Design review of the part built by this model. Coordinates are the model's own, in mm. A direction names the side the tool comes from. Give positions to 0.01 mm unless a question says otherwise; leave off trailing zeros. Loops run counter-clockwise (first coordinate to the right, second up) from the corner with the lowest first, then second, coordinate; pieces in that order, holes last. Notation, with made-up numbers: (-35, 29) - (-28, 29) arc R23 cw to (-28, 53) - close; hole circle Ø1 at (89, 63.25). An arc over 180 degrees is marked (long way). Write each question's results on one line, items separated by ' | '.
from build123d import *
from build123d.topology import SkipClean

# Parameters (mm, degrees)
EXTRUDE_1_DEPTH        = 4
EXTRUDE_3_DEPTH        = 6
CHAMFER_1_SIZE         = 3
SKETCH_5_R             = 0.85
CUT_EXTRUDE_1_DEPTH    = 4
PATTERN_LINEAR_1_COUNT = 4
PATTERN_LINEAR_1_PITCH = 8
CUT_EXTRUDE_2_DEPTH    = 2.5
CUT_EXTRUDE_3_REACH    = 41.439
SKETCH_7_R             = 1.35
SKETCH_8_R             = 6
EXTRUDE_4_DEPTH        = 1.5
FILLET_1_R             = 0.5
SKETCH_9_R             = 5
CUT_EXTRUDE_4_DEPTH    = 3.6
SKETCH_10_R            = 3.55
CUT_EXTRUDE_5_DEPTH    = 3.6
CUT_EXTRUDE_6_DEPTH    = 0.8
CUT_EXTRUDE_7_DEPTH    = 40.958228189
FILLET_2_R             = 2
CHAMFER_2_SIZE         = 1


with BuildPart() as part:
    # ｽｹｯﾁ1 → ﾎﾞｽ - 押し出し1 (new body)
    with BuildSketch(Plane(origin=(0, 0, 0), x_dir=(1, 0, 0), z_dir=(0, 1, 0))):
        with BuildLine():
            Line((-7.9, 0), (-7.9, -38))
            Line((-7.9, -38), (7.9, -38))
            Line((7.9, -38), (7.9, 0))
            ThreePointArc((7.9, 0), (0, 7.9), (-7.9, 0))
        make_face()
    extrude(amount=EXTRUDE_1_DEPTH)

    # ｽｹｯﾁ4 → ﾎﾞｽ - 押し出し3 (add)
    with BuildSketch(Plane.XY.offset(38)):
        Polygon((-7, -5.5), (-4.5, -5.5), (-3, -2), (3, -2), (4.5, -5.5), (7, -5.5), (7.9, -2), (7.9, 0), (-7.9, 0), (-7.9, -2), align=None)
    extrude(amount=-EXTRUDE_3_DEPTH)

    # 面取り1
    chamfer_1_edges = [part.edges().sort_by_distance(p)[0] for p in [
        (0, 4, 38),
    ]]
    chamfer(chamfer_1_edges, length=CHAMFER_1_SIZE)

    # ｽｹｯﾁ5 → ｶｯﾄ - 押し出し1 (cut)
    with BuildSketch(Plane(origin=(0, 4, 0), x_dir=(1, 0, 0), z_dir=(0, 1, 0))):
        with Locations(Location((-4, -31, 0), (0, 0, 270))):
            Circle(SKETCH_5_R)
        with Locations(Location((4, -31, 0), (0, 0, 270))):
            Circle(SKETCH_5_R)
    cut_extrude_1 = extrude(amount=-CUT_EXTRUDE_1_DEPTH, mode=Mode.SUBTRACT)

    # 直線ﾊﾟﾀｰﾝ1: ｶｯﾄ - 押し出し1 ×4
    with Locations(*[(0, 0, -i * PATTERN_LINEAR_1_PITCH) for i in range(1, PATTERN_LINEAR_1_COUNT)]):
        add(cut_extrude_1, mode=Mode.SUBTRACT)

    # ｽｹｯﾁ6 → ｶｯﾄ - 押し出し2 (cut)
    with BuildSketch(Plane(origin=(0, 4, 0), x_dir=(1, 0, 0), z_dir=(0, 1, 0))):
        with BuildLine():
            Line((-3, -35), (-3, -39))
            Line((-3, -39), (3, -39))
            Line((3, -39), (3, -35))
            ThreePointArc((3, -35), (0, -32), (-3, -35))
        make_face()
    extrude(amount=-CUT_EXTRUDE_2_DEPTH, mode=Mode.SUBTRACT)

    # ｽｹｯﾁ7 → ｶｯﾄ - 押し出し3 (cut, up to next)
    with BuildSketch(Plane(origin=(0, 1.5, 0), x_dir=(1, 0, 0), z_dir=(0, 1, 0)), mode=Mode.PRIVATE) as cut_extrude_3_sk1:
        with Locations(Location((0, -35, 0), (0, 0, 270))):
            Circle(SKETCH_7_R)
    cut_extrude_3_tool1 = extrude(cut_extrude_3_sk1.sketch, amount=-CUT_EXTRUDE_3_REACH, mode=Mode.PRIVATE) & part.part
    add(cut_extrude_3_tool1.solids().sort_by_distance((0, 1.5, 35))[0], mode=Mode.SUBTRACT)

    # ｽｹｯﾁ8 → ﾎﾞｽ - 押し出し4 (add)
    with BuildSketch(Plane.XZ):
        with Locations(Location((0, 0, 0), (0, 0, 90))):
            Circle(SKETCH_8_R)
    extrude(amount=EXTRUDE_4_DEPTH)

    # ﾌｨﾚｯﾄ1
    fillet_1_edges = [part.edges().sort_by_distance(p)[0] for p in [
        (0, 0, -6),
    ]]
    fillet(fillet_1_edges, radius=FILLET_1_R)

    # ｽｹｯﾁ9 → ｶｯﾄ - 押し出し4 (cut)
    with BuildSketch(Plane(origin=(0, 4, 0), x_dir=(1, 0, 0), z_dir=(0, 1, 0))):
        with Locations(Location((0, 0, 0), (0, 0, 270))):
            Circle(SKETCH_9_R)
    extrude(amount=-CUT_EXTRUDE_4_DEPTH, mode=Mode.SUBTRACT)

    # ｽｹｯﾁ10 → ｶｯﾄ - 押し出し5 (cut)
    with BuildSketch(Plane(origin=(0, 0.4, 0), x_dir=(1, 0, 0), z_dir=(0, 1, 0))):
        with Locations(Location((0, 0, 0), (0, 0, 270))):
            Circle(SKETCH_10_R)
    extrude(amount=-CUT_EXTRUDE_5_DEPTH, mode=Mode.SUBTRACT)

    # ｽｹｯﾁ11 → ｶｯﾄ - 押し出し6 (cut, symmetric)
    with BuildSketch(Plane.XY.offset(35)):
        Polygon((3, -2), (4.5, -5.5), (5.1, -5.5), (3.6, -2), align=None)
        Polygon((7.9, -2), (7, -5.5), (6.4, -5.5), (7.3, -2), align=None)
    cut_extrude_6 = extrude(amount=CUT_EXTRUDE_6_DEPTH, both=True, mode=Mode.SUBTRACT)

    # ﾐﾗｰ1: ｶｯﾄ - 押し出し6 across plane
    add(cut_extrude_6.mirror(Plane(origin=(0, 0, 0), x_dir=(0, 0, 1), z_dir=(1, 0, 0))), mode=Mode.SUBTRACT)

    # ｽｹｯﾁ12 → ｶｯﾄ - 押し出し7 (cut, through all)
    with SkipClean():  # the faces are left unmerged after this step: merging them gives an invalid solid
        with BuildSketch(Plane(origin=(0, 4, 0), x_dir=(1, 0, 0), z_dir=(0, 1, 0))):
            with BuildLine():
                Line((-7.9, 0), (-7.9, -30))
                Line((-7.9, -30), (-6.9, -27))
                Line((-6.9, -27), (-6.9, -3.847076812))
                ThreePointArc((-6.9, -3.847076812), (-7.645913941, -1.987460691), (-7.9, 0))
            make_face()
        cut_extrude_7 = extrude(amount=-CUT_EXTRUDE_7_DEPTH, mode=Mode.SUBTRACT)

    # ﾐﾗｰ2: ｶｯﾄ - 押し出し7 across plane
    with SkipClean():  # the faces are left unmerged after this step: merging them gives an invalid solid
        add(cut_extrude_7.mirror(Plane(origin=(0, 0, 0), x_dir=(0, 0, 1), z_dir=(1, 0, 0))), mode=Mode.SUBTRACT)

    # ﾌｨﾚｯﾄ2
    fillet_2_edges = [part.edges().sort_by_distance(p)[0] for p in [
        (-6.9, 2, 3.847076812),
        (-6.9, 2, 27),
        (-7.9, 2, 30),
        (6.9, 2, 3.847076812),
        (7.9, 2, 30),
        (6.9, 2, 27),
    ]]
    fillet(fillet_2_edges, radius=FILLET_2_R)

    # 面取り2
    # the kernel refuses this chamfer: 1 mm, written as the material it adds along each edge
    with BuildSketch(Plane(origin=(7.9, 0, 32), x_dir=(0, 0.02749587661058639, -0.9996219169112968), z_dir=(-1, 0, 0))) as chamfer_2_piece_1_section:
        Polygon((CHAMFER_2_SIZE * 0.999621916911, CHAMFER_2_SIZE * 0.0274958766106), (-CHAMFER_2_SIZE * 0.0274958766106, CHAMFER_2_SIZE * 0.999621916911), (0, 0), align=None)
    chamfer_2_piece_1 = extrude(amount=15.8, mode=Mode.PRIVATE)
    chamfer_2_piece_1 = chamfer_2_piece_1 - Plane(origin=(-4, -0.34097177, 31), x_dir=(0, 0, 1), z_dir=(0, 1, 0)) * Cylinder(0.85, 36, mode=Mode.PRIVATE)
    chamfer_2_piece_1 = chamfer_2_piece_1 - Plane(origin=(4, -0.34097177, 31), x_dir=(0, 0, 1), z_dir=(0, 1, 0)) * Cylinder(0.85, 36, mode=Mode.PRIVATE)
    add(chamfer_2_piece_1)
    # the kernel refuses this chamfer: 1 mm, written as the material it takes off along each edge
    with BuildSketch(Plane(origin=(-7.9, 4, 30.32455532), x_dir=(-0.027495876610586487, -0.9996219169112968, 0), z_dir=(0, 0, 1)), Plane(origin=(7.9, 4, 37.571682988), x_dir=(0.027495876610586487, -0.9996219169112968, 0), z_dir=(0, 0, -1))) as chamfer_2_2_piece_1:
        Polygon((CHAMFER_2_SIZE * 0.999621916911, CHAMFER_2_SIZE * 0.0274958766106), (-CHAMFER_2_SIZE * 0.0274958766106, CHAMFER_2_SIZE * 0.999621916911), (0, 0), align=None)
    extrude(amount=7.247127668, mode=Mode.SUBTRACT)
    with BuildSketch(Plane(origin=(0, 4, 0), x_dir=(1, 0, 0), z_dir=(0, 0, 1))) as chamfer_2_2_piece_2:
        Polygon((7.9, -CHAMFER_2_SIZE), (7.9 - CHAMFER_2_SIZE, 0), (7.9, 0), align=None)
    revolve(axis=Axis((0, 4, 0), (0, 1, 0)), revolution_arc=180, mode=Mode.SUBTRACT)
    with BuildSketch(Plane(origin=(-5.9, 4, 30.32455532), x_dir=(-1, 0, 0), z_dir=(0, 0, 1))) as chamfer_2_2_piece_3:
        Polygon((2, CHAMFER_2_SIZE), (2 - CHAMFER_2_SIZE, 0), (2, 0), align=None)
    revolve(axis=Axis((-5.9, 4, 30.32455532), (0, -1, 0)), revolution_arc=18.434948823, mode=Mode.SUBTRACT)
    with BuildSketch(Plane(origin=(-7.797366596, 4, 29.692099788), x_dir=(-0.02608487890572092, -0.9996219169112968, -0.008694959635240314), z_dir=(0.3162277660168382, 0, -0.9486832980505138))) as chamfer_2_2_piece_4:
        Polygon((CHAMFER_2_SIZE * 0.999621916911, -CHAMFER_2_SIZE * 0.0274958766106), (-CHAMFER_2_SIZE * 0.0274958766106, -CHAMFER_2_SIZE * 0.999621916911), (0, 0), align=None)
    extrude(amount=2.513167019, mode=Mode.SUBTRACT)
    with BuildSketch(Plane(origin=(-8.9, 4, 26.67544468), x_dir=(0.9486832980505135, 0, 0.3162277660168389), z_dir=(-0.3162277660168389, 0, 0.9486832980505135))) as chamfer_2_2_piece_5:
        Polygon((2, -CHAMFER_2_SIZE), (2 + CHAMFER_2_SIZE, 0), (2, 0), align=None)
    revolve(axis=Axis((-8.9, 4, 26.67544468), (0, 1, 0)), revolution_arc=18.434948823, mode=Mode.SUBTRACT)
    with BuildSketch(Plane(origin=(-6.9, 4, 26.67544468), x_dir=(-0.027495876610586487, -0.9996219169112968, 0), z_dir=(0, 0, -1))) as chamfer_2_2_piece_6:
        Polygon((CHAMFER_2_SIZE * 0.999621916911, -CHAMFER_2_SIZE * 0.0274958766106), (-CHAMFER_2_SIZE * 0.0274958766106, -CHAMFER_2_SIZE * 0.999621916911), (0, 0), align=None)
    extrude(amount=22.339548002, mode=Mode.SUBTRACT)
    with BuildSketch(Plane(origin=(-8.9, 4, 4.335896678), x_dir=(1, 0, 0), z_dir=(0, 0, 1))) as chamfer_2_2_piece_7:
        Polygon((2, -CHAMFER_2_SIZE), (2 + CHAMFER_2_SIZE, 0), (2, 0), align=None)
    revolve(axis=Axis((-8.9, 4, 4.335896678), (0, 1, 0)), revolution_arc=25.974390018, mode=Mode.SUBTRACT)
    with BuildSketch(Plane(origin=(8.9, 4, 4.335896678), x_dir=(-0.8989898989898989, 0, -0.43796936138745074), z_dir=(0.43796936138745074, 0, -0.8989898989898989))) as chamfer_2_2_piece_8:
        Polygon((2, -CHAMFER_2_SIZE), (2 + CHAMFER_2_SIZE, 0), (2, 0), align=None)
    revolve(axis=Axis((8.9, 4, 4.335896678), (0, 1, 0)), revolution_arc=25.974390018, mode=Mode.SUBTRACT)
    with BuildSketch(Plane(origin=(6.9, 4, 26.67544468), x_dir=(0.027495876610586487, -0.9996219169112968, 0), z_dir=(0, 0, -1))) as chamfer_2_2_piece_9:
        Polygon((CHAMFER_2_SIZE * 0.999621916911, CHAMFER_2_SIZE * 0.0274958766106), (-CHAMFER_2_SIZE * 0.0274958766106, CHAMFER_2_SIZE * 0.999621916911), (0, 0), align=None)
    extrude(amount=22.339548002, mode=Mode.SUBTRACT)
    with BuildSketch(Plane(origin=(8.9, 4, 26.67544468), x_dir=(-1, 0, 0), z_dir=(0, 0, -1))) as chamfer_2_2_piece_10:
        Polygon((2, -CHAMFER_2_SIZE), (2 + CHAMFER_2_SIZE, 0), (2, 0), align=None)
    revolve(axis=Axis((8.9, 4, 26.67544468), (0, 1, 0)), revolution_arc=18.434948823, mode=Mode.SUBTRACT)
    with BuildSketch(Plane(origin=(7.797366596, 4, 29.692099788), x_dir=(0.02608487890572092, -0.9996219169112968, -0.008694959635240314), z_dir=(-0.3162277660168382, 0, -0.9486832980505138))) as chamfer_2_2_piece_11:
        Polygon((CHAMFER_2_SIZE * 0.999621916911, CHAMFER_2_SIZE * 0.0274958766106), (-CHAMFER_2_SIZE * 0.0274958766106, CHAMFER_2_SIZE * 0.999621916911), (0, 0), align=None)
    extrude(amount=2.513167019, mode=Mode.SUBTRACT)
    with BuildSketch(Plane(origin=(5.9, 4, 30.32455532), x_dir=(0.9486832980505135, 0, -0.3162277660168389), z_dir=(-0.3162277660168389, 0, -0.9486832980505135))) as chamfer_2_2_piece_12:
        Polygon((2, CHAMFER_2_SIZE), (2 - CHAMFER_2_SIZE, 0), (2, 0), align=None)
    revolve(axis=Axis((5.9, 4, 30.32455532), (0, -1, 0)), revolution_arc=18.434948823, mode=Mode.SUBTRACT)
    with BuildSketch(Plane(origin=(0, 4, 0), x_dir=(0.8989898989898987, 0, 0.43796936138745124), z_dir=(-0.43796936138745124, 0, 0.8989898989898987))) as chamfer_2_2_piece_13:
        Polygon((7.9, -CHAMFER_2_SIZE), (7.9 - CHAMFER_2_SIZE, 0), (7.9, 0), align=None)
    revolve(axis=Axis((0, 4, 0), (0, 1, 0)), revolution_arc=25.974390018, mode=Mode.SUBTRACT)
    with BuildSketch(Plane(origin=(0, 4, 0), x_dir=(-0.8989898989898987, 0, 0.43796936138745124), z_dir=(0.43796936138745124, 0, 0.8989898989898987))) as chamfer_2_2_piece_14:
        Polygon((7.9, CHAMFER_2_SIZE), (7.9 - CHAMFER_2_SIZE, 0), (7.9, 0), align=None)
    revolve(axis=Axis((0, 4, 0), (0, -1, 0)), revolution_arc=25.974390018, mode=Mode.SUBTRACT)


solid = part.part
(1) Insertion check: P1, Ø3.5, axis at y = 1.5, z = 20.5, coming from the -X side; P2, Ø2, axis at x = -4, y = 0.5, coming from the -Z side; P3, Ø0.6, axis at x = -4, y = -4.5, coming from the -Z side; P4, Ø1.4, axis at x = 4, z = 31, coming from the +Y side. Each pin has a flat end and moves straight along its axis. Give the tip position at first contact, or say it passes through.
Answers below:
P1: x = -6.9 | P2: z = -7.31 | P3: z = 32 | P4: through
(2) Take a section at A-A on y = -3.75. Give the boundary of the cut face in (x, z).
Answers below:
outline: (-7.45, 32) - (-3.75, 32) - (-3.75, 34.2) - (-4.35, 34.2) - (-4.35, 35.8) - (-3.75, 35.8) - (-3.75, 38) - (-7.45, 38) - (-7.45, 35.8) - (-6.85, 35.8) - (-6.85, 34.2) - (-7.45, 34.2) - close; (3.75, 32) - (7.45, 32) - (7.45, 34.2) - (6.85, 34.2) - (6.85, 35.8) - (7.45, 35.8) - (7.45, 38) - (3.75, 38) - (3.75, 35.8) - (4.35, 35.8) - (4.35, 34.2) - (3.75, 34.2) - close
(3) Draft analysis for pull direction Z (two halves, no side actions). For faces 1 (the flat face through (3.74, -3.73, 33.12)), 2 (the conical face through (-6.426, 3.507, 27.083)), 3 (the flat face through (0, -1, 38)), state which applies: pulls with the +Z half, pulls with the -Z half, needs draft (parallel to the pull), parting line crosses it, or undercut.
Answers below:
face 1: needs draft | face 2: undercut | face 3: pulls with the +Z half
(4) Take a section at B-B on y = 2.5. Count the separate pieces of the cut face and the enclosed holes in it, plus the area to 3 significant figures.
Answers below:
separate pieces: 1 | enclosed holes: 9 | area: 503 mm2
(5) Tool access review of faces 4 (the conical face through (7.37, 3.51, 30.08)), 5 (the flat face through (-4, -3.7, 35.8)), 6 (the flat face through (3, -1.5, 3)), 7 (the flat face through (0, 1.5, 33)), 8 (the flat face through (-6.9, 2, 16)): name each direction out of +Z, -Z, +X, -X, +Y, -Y from which nothing blocks a thin tool from reaching the whole face with its end or side.
Answers below:
face 4: +X, +Y | face 5: -Y | face 6: -Z, +X, -X, -Y | face 7: +Z, +Y | face 8: -X, +Y, -Y
(6) Wall thickness on line 1 along X through (y, z) = (2.7, 15); line 2 along X through (y, z) = (0.25, 31); line 3 along Z through (x, y) = (-4.5, -4.5): over which ranges is each line inside the solid? List them lowest first. Write a range as from..to.
Answers below:
line 1: -6.9..-4.85, -3.15..3.15, 4.85..6.9 | line 2: -7.9..-4.85, -3.15..3.15, 4.85..7.9 | line 3: 32..34.2, 35.8..38
(7) Take a section at D-D on z = 23. Give the boundary of the cut face in (x, y).
Answers below:
outline: (-6.9, 0) - (-4.85, 0) - (-4.85, 4) - (-5.9, 4) - (-6.9, 3) - close; (-3.15, 0) - (3.15, 0) - (3.15, 4) - (-3.15, 4) - close; (4.85, 0) - (6.9, 0) - (6.9, 3) - (5.9, 4) - (4.85, 4) - close
